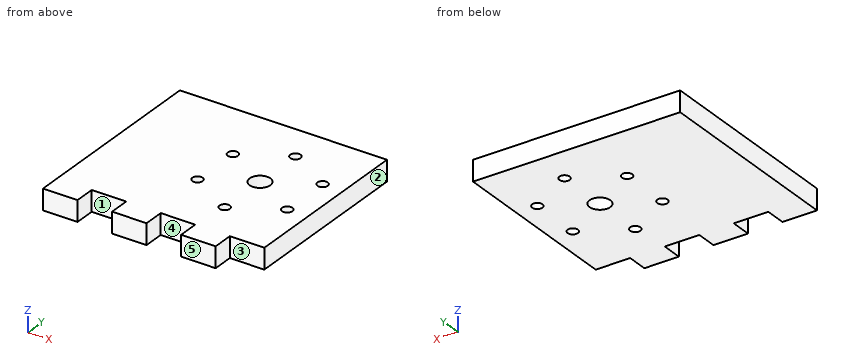
from build123d import *

# Parameters (mm, degrees)
SKETCH1_R             = 0.75
SKETCH1_R_2           = 1.5
BOSS_EXTRUDE1_DEPTH   = 3
CORTAR_EXTRUIR1_START = -3
CROQUIS1_W            = 15
CROQUIS1_H            = 6.71890751
CORTAR_EXTRUIR1_DEPTH = 3


with BuildPart() as part:
    # Sketch1 → Boss-Extrude1 (new body)
    with BuildSketch(Plane.XY):
        Polygon((10, 0), (10, 3), (15, 3), (15, 0), (20, 0), (20, 3), (25, 3), (25, 0), (30, 0), (30, -26), (25, -26), (25, -29), (20, -29), (20, -26), (15, -26), (15, -29), (10, -29), (10, -26), (5, -26), (5, -29), (0, -29), (0, 0), align=None)
        with Locations((20.5, -5.5)):
            Circle(SKETCH1_R, mode=Mode.SUBTRACT)
        with Locations((26.995190528, -9.25)):
            Circle(SKETCH1_R, mode=Mode.SUBTRACT)
        with Locations((26.995190528, -16.75)):
            Circle(SKETCH1_R, mode=Mode.SUBTRACT)
        with Locations((20.5, -20.5)):
            Circle(SKETCH1_R, mode=Mode.SUBTRACT)
        with Locations((14.004809472, -16.75)):
            Circle(SKETCH1_R, mode=Mode.SUBTRACT)
        with Locations((14.004809472, -9.25)):
            Circle(SKETCH1_R, mode=Mode.SUBTRACT)
        with Locations((20.5, -13)):
            Circle(SKETCH1_R_2, mode=Mode.SUBTRACT)
    extrude(amount=BOSS_EXTRUDE1_DEPTH)

    # Croquis1 → Cortar-Extruir1 (cut)
    with BuildSketch(Plane.XY.offset(3).offset(CORTAR_EXTRUIR1_START)):
        with Locations((17.5, 3.359453755)):
            Rectangle(CROQUIS1_W, CROQUIS1_H)
    extrude(amount=CORTAR_EXTRUIR1_DEPTH, mode=Mode.SUBTRACT)


solid = part.part
Geometry check sheet. Reference: the model listing, model coordinates, mm. Face numbers are marked on the shaded views. A direction names the side the tool comes from. Give positions to 0.01 mm unless a question says otherwise; leave off trailing zeros. Loops run counter-clockwise (first coordinate to the right, second up) from the corner with the lowest first, then second, coordinate; pieces in that order, holes last.
(1) Set-up check for the marked faces 4 and 5: record each of +Z, -Z, +X, -X, +Y, -Y from which the full face is reachable in a straight line by a thin tool's end or side.
From the geometry:
face 4: +Z, -Z, -Y
face 5: +Z, -Z, +X, -X, -Y
(2) Section check D-D on x = 18.5. Record the cut outline in (y, z), then the cut area to 3 significant figures.
From the geometry:
outline: (-26, 0) - (0, 0) - (0, 3) - (-26, 3) - close
area: 78.0 mm2
(3) Thickness scan on L1, parallel to Y at x = 20.5, z = 2.15; L2, parallel to Y at x = 27.5, z = 2.2; L3, parallel to Y at x = 28.25, z = 0.5. Record the ranges inside material, lowest first.
From the geometry:
L1: y = -29 to -21.25, -19.75 to -14.5, -11.5 to -6.25, -4.75 to 0
L2: y = -26 to -17.3, -16.2 to -9.8, -8.7 to 0
L3: y = -26 to 0
(4) Section check C-C on z = 2.4. Record the cut outline in (x, y).
From the geometry:
outline: (0, -29) - (5, -29) - (5, -26) - (10, -26) - (10, -29) - (15, -29) - (15, -26) - (20, -26) - (20, -29) - (25, -29) - (25, -26) - (30, -26) - (30, 0) - (0, 0) - close; hole circle Ø1.5 at (14, -16.75); hole circle Ø1.5 at (14, -9.25); hole circle Ø3 at (20.5, -13); hole circle Ø1.5 at (20.5, -20.5); hole circle Ø1.5 at (20.5, -5.5); hole circle Ø1.5 at (27, -16.75); hole circle Ø1.5 at (27, -9.25)
(5) Section check A-A on y = -20.5. Record the cut outline in (x, z), then the cut area to 3 significant figures.
From the geometry:
outline: (0, 0) - (19.75, 0) - (19.75, 3) - (0, 3) - close; (21.25, 0) - (30, 0) - (30, 3) - (21.25, 3) - close
area: 85.5 mm2
(6) Depth check by flat-ended pin: pin 1 Ø0.9 at (y, z) = (-27, 1) entering from -X; pin 2 Ø1.5 at (y, z) = (-28, 1.5) entering from +X; pin 3 Ø1.5 at (x, z) = (7, 2) entering from -Y. Enter the tip coordinate at first touch or a pass-through.
From the geometry:
pin 1: stops at x = 0
pin 2: stops at x = 25
pin 3: stops at y = -26
(7) Release check for a two-part mould opening along X. For the marked faces 1, 2 and 3 record: released by +X, released by -X, zero draft, split by the parting line, or undercut.
From the geometry:
face 1: undercut
face 2: released by +X
face 3: zero draft
(8) Section check B-B on y = -16.75. Record the cut outline in (x, z).
From the geometry:
outline: (0, 0) - (13.25, 0) - (13.25, 3) - (0, 3) - close; (14.75, 0) - (26.25, 0) - (26.25, 3) - (14.75, 3) - close; (27.75, 0) - (30, 0) - (30, 3) - (27.75, 3) - close
